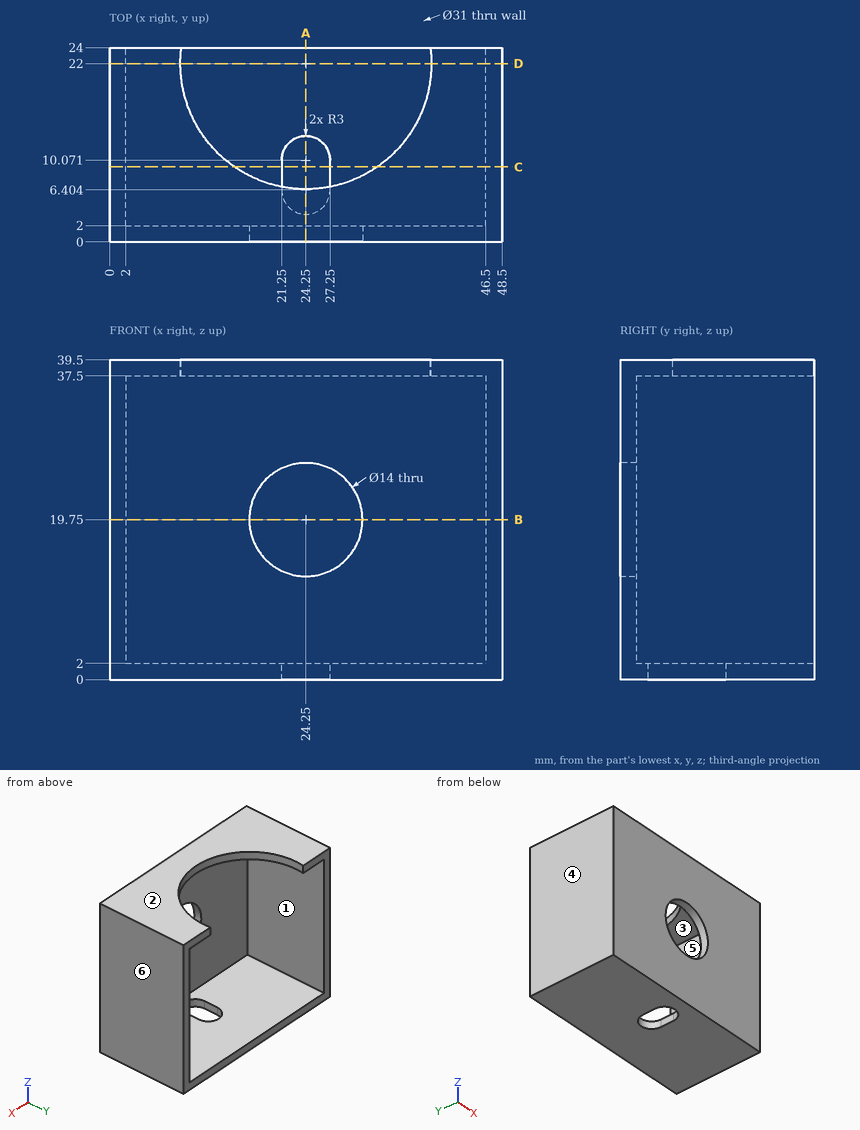
Verification items for this drawing (mm, ordinates from the low corner). A direction names the side the tool comes from. Give positions to 0.01 mm unless a question says otherwise; leave off trailing zeros. Order: outer loops, then holes, each group sorted by start corner. A loop starts at its lowest first (then second) coordinate and runs counter-clockwise, first axis right, second up. Notation, with made-up numbers: M -6,35.25 L 49,35.25 A20 cw 49,58.25 Z; hole C 49,82 d9. An arc over 180 degrees is marked long. Use a Markdown table: item, result.
Item 1: Depth check by flat-ended pin: P1, Ø6.5, axis at x = 19, y = 14, coming from the +Z side. Enter the tip coordinate at first touch or a pass-through.
Answers follow:
| item | result |
|---|---|
| P1 | stops at z = 2 |
Item 2: Section check B-B (z = 19.75). Record the cut outline in (x, y), and give its area (3 significant figures).
Answers follow:
| item | result |
|---|---|
| outline | M 0,0 L 17.25,0 L 17.25,2 L 2,2 L 2,24 L 0,24 Z; M 31.25,0 L 48.5,0 L 48.5,24 L 46.5,24 L 46.5,2 L 31.25,2 Z |
| area | 157 mm2 |
Item 3: Material ranges on line 1 along X through (y, z) = (1.65, 19.75); line 2 along X through (y, z) = (21.5, 8); line 3 along Z through (x, y) = (11, 13.5), recorded low to high.
Answers follow:
| item | result |
|---|---|
| line 1 | x = 0 to 17.25, 31.25 to 48.5 |
| line 2 | x = 0 to 2, 46.5 to 48.5 |
| line 3 | z = 0 to 2, 37.5 to 39.5 |
Item 4: Tool access check on the marked faces 5 and 6. Record the directions out of +Z, -Z, +X, -X, +Y, -Y that give a thin tool (end or side, any length) a straight path to the whole face; none if there is none.
Answers follow:
| item | result |
|---|---|
| face 5 | +Y |
| face 6 | +Z, -Z, +X, +Y, -Y |
Item 5: Section check D-D (y = 22). Record the cut outline in (x, z), and give its area (3 significant figures).
Answers follow:
| item | result |
|---|---|
| outline | M 0,0 L 48.5,0 L 48.5,39.5 L 39.75,39.5 L 39.75,37.5 L 46.5,37.5 L 46.5,2 L 2,2 L 2,37.5 L 8.75,37.5 L 8.75,39.5 L 0,39.5 Z |
| area | 274 mm2 |
Item 6: Draft check along Z on the marked faces 1, 2, 3 and 4. Enter one of: +Z half, -Z half, draft (parallel to the pull), parting line (faces both ways), or undercut.
Answers follow:
| item | result |
|---|---|
| face 1 | undercut |
| face 2 | +Z half |
| face 3 | undercut |
| face 4 | draft |
Item 7: Section check C-C (y = 9.25). Record the cut outline in (x, z), and give its area (3 significant figures).
Answers follow:
| item | result |
|---|---|
| outline | M 0,0 L 21.25,0 L 21.25,2 L 2,2 L 2,37.5 L 15.44,37.5 L 15.44,39.5 L 0,39.5 Z; M 27.25,0 L 48.5,0 L 48.5,39.5 L 33.06,39.5 L 33.06,37.5 L 46.5,37.5 L 46.5,2 L 27.25,2 Z |
| area | 289 mm2 |
Item 8: Section check A-A (x = 24.25). Record the cut outline in (y, z).
Answers follow:
| item | result |
|---|---|
| outline | M 0,0 L 3.4,0 L 3.4,2 L 2,2 L 2,12.75 L 0,12.75 Z; M 0,26.75 L 2,26.75 L 2,37.5 L 6.5,37.5 L 6.5,39.5 L 0,39.5 Z; M 13.07,0 L 24,0 L 24,2 L 13.07,2 Z |
